```python
from build123d import *

# Parameters (mm, degrees)
SZKIC1_R                    = 2.25
DODANIE_WYCI_GNI_CIE1_DEPTH = 4


with BuildPart() as part:
    # Szkic1 → Dodanie-wyciągnięcie1 (new body)
    with BuildSketch(Plane.XY):
        with BuildLine():
            Line((-0.65, 5.460113222), (-0.65, 4.452808103))
            ThreePointArc((-0.65, 4.452808103), (-1.076920489, 4.369238178), (-1.493776689, 4.244835827))
            Line((-1.493776689, 4.244835827), (-1.96189472, 5.136760215))
            Line((-1.96189472, 5.136760215), (-2.706408708, 5.9097675))
            Line((-2.706408708, 5.9097675), (-3.326227926, 5.58446128))
            Line((-3.326227926, 5.58446128), (-3.112987553, 4.532620091))
            Line((-3.112987553, 4.532620091), (-2.644869523, 3.640695704))
            ThreePointArc((-2.644869523, 3.640695704), (-2.984051962, 3.368298367), (-3.295347141, 3.06442282))
            Line((-3.295347141, 3.06442282), (-4.124343002, 3.636637347))
            Line((-4.124343002, 3.636637347), (-5.142811797, 3.975108403))
            Line((-5.142811797, 3.975108403), (-5.54045712, 3.399019697))
            Line((-5.54045712, 3.399019697), (-4.862827173, 2.566758322))
            Line((-4.862827173, 2.566758322), (-4.033831312, 1.994543794))
            ThreePointArc((-4.033831312, 1.994543794), (-4.207573092, 1.595721992), (-4.341993276, 1.181987475))
            Line((-4.341993276, 1.181987475), (-5.341954007, 1.30340469))
            Line((-5.341954007, 1.30340469), (-6.401058681, 1.129799877))
            Line((-6.401058681, 1.129799877), (-6.485434357, 0.434903665))
            Line((-6.485434357, 0.434903665), (-5.498651691, 0.012883153))
            Line((-5.498651691, 0.012883153), (-4.49869096, -0.108534062))
            ThreePointArc((-4.49869096, -0.108534062), (-4.467189933, -0.542415061), (-4.393941078, -0.971226957))
            Line((-4.393941078, -0.971226957), (-5.335787726, -1.328422275))
            Line((-5.335787726, -1.328422275), (-6.192900162, -1.974332186))
            Line((-6.192900162, -1.974332186), (-5.944676741, -2.628843556))
            Line((-5.944676741, -2.628843556), (-4.874801373, -2.54394339))
            Line((-4.874801373, -2.54394339), (-3.932954725, -2.186748072))
            ThreePointArc((-3.932954725, -2.186748072), (-3.703427397, -2.55629136), (-3.439289932, -2.901944997))
            Line((-3.439289932, -2.901944997), (-4.10725678, -3.655923705))
            Line((-4.10725678, -3.655923705), (-4.566022849, -4.626168538))
            Line((-4.566022849, -4.626168538), (-4.042065325, -5.090354399))
            Line((-4.042065325, -5.090354399), (-3.134192808, -4.517983161))
            Line((-3.134192808, -4.517983161), (-2.466225959, -3.764004452))
            ThreePointArc((-2.466225959, -3.764004452), (-2.091254274, -3.984552115), (-1.69673891, -4.16786241))
            Line((-1.69673891, -4.16786241), (-1.937802804, -5.145897073))
            Line((-1.937802804, -5.145897073), (-1.893124727, -6.21820543))
            Line((-1.893124727, -6.21820543), (-1.213465455, -6.385726395))
            Line((-1.213465455, -6.385726395), (-0.675578441, -5.457007437))
            Line((-0.675578441, -5.457007437), (-0.434514548, -4.478972774))
            ThreePointArc((-0.434514548, -4.478972774), (0, -4.5), (0.434514548, -4.478972774))
            Line((0.434514548, -4.478972774), (0.675578441, -5.457007437))
            Line((0.675578441, -5.457007437), (1.213465455, -6.385726395))
            Line((1.213465455, -6.385726395), (1.893124727, -6.21820543))
            Line((1.893124727, -6.21820543), (1.937802804, -5.145897073))
            Line((1.937802804, -5.145897073), (1.69673891, -4.16786241))
            ThreePointArc((1.69673891, -4.16786241), (2.091254274, -3.984552115), (2.466225959, -3.764004452))
            Line((2.466225959, -3.764004452), (3.134192808, -4.517983161))
            Line((3.134192808, -4.517983161), (4.042065325, -5.090354399))
            Line((4.042065325, -5.090354399), (4.566022849, -4.626168538))
            Line((4.566022849, -4.626168538), (4.10725678, -3.655923705))
            Line((4.10725678, -3.655923705), (3.439289932, -2.901944997))
            ThreePointArc((3.439289932, -2.901944997), (3.703427397, -2.55629136), (3.932954725, -2.186748072))
            Line((3.932954725, -2.186748072), (4.874801373, -2.54394339))
            Line((4.874801373, -2.54394339), (5.944676741, -2.628843556))
            Line((5.944676741, -2.628843556), (6.192900162, -1.974332186))
            Line((6.192900162, -1.974332186), (5.335787726, -1.328422275))
            Line((5.335787726, -1.328422275), (4.393941078, -0.971226957))
            ThreePointArc((4.393941078, -0.971226957), (4.467189933, -0.542415061), (4.49869096, -0.108534062))
            Line((4.49869096, -0.108534062), (5.498651691, 0.012883153))
            Line((5.498651691, 0.012883153), (6.485434357, 0.434903665))
            Line((6.485434357, 0.434903665), (6.401058681, 1.129799877))
            Line((6.401058681, 1.129799877), (5.341954007, 1.30340469))
            Line((5.341954007, 1.30340469), (4.341993276, 1.181987475))
            ThreePointArc((4.341993276, 1.181987475), (4.207573092, 1.595721992), (4.033831312, 1.994543794))
            Line((4.033831312, 1.994543794), (4.862827173, 2.566758322))
            Line((4.862827173, 2.566758322), (5.54045712, 3.399019697))
            Line((5.54045712, 3.399019697), (5.142811797, 3.975108403))
            Line((5.142811797, 3.975108403), (4.124343002, 3.636637347))
            Line((4.124343002, 3.636637347), (3.295347141, 3.06442282))
            ThreePointArc((3.295347141, 3.06442282), (2.984051962, 3.368298367), (2.644869523, 3.640695704))
            Line((2.644869523, 3.640695704), (3.112987553, 4.532620091))
            Line((3.112987553, 4.532620091), (3.326227926, 5.58446128))
            Line((3.326227926, 5.58446128), (2.706408708, 5.9097675))
            Line((2.706408708, 5.9097675), (1.96189472, 5.136760215))
            Line((1.96189472, 5.136760215), (1.493776689, 4.244835827))
            ThreePointArc((1.493776689, 4.244835827), (1.076920489, 4.369238178), (0.65, 4.452808103))
            Line((0.65, 4.452808103), (0.65, 5.460113222))
            Line((0.65, 5.460113222), (0.35, 6.490570083))
            Line((0.35, 6.490570083), (-0.35, 6.490570083))
            Line((-0.35, 6.490570083), (-0.65, 5.460113222))
        make_face()
        Circle(SZKIC1_R, mode=Mode.SUBTRACT)
    extrude(amount=DODANIE_WYCI_GNI_CIE1_DEPTH)


solid = part.part
```
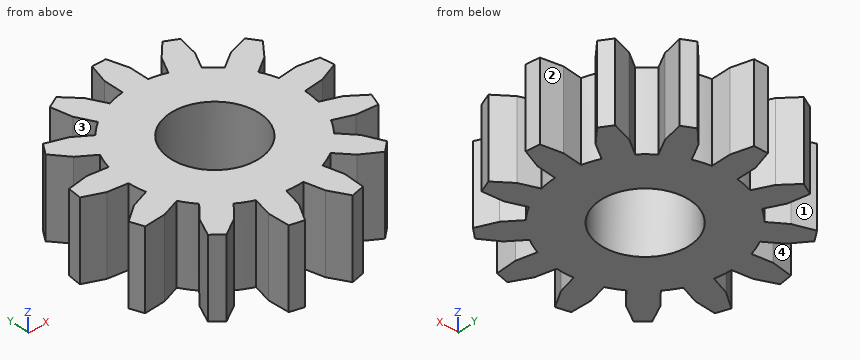
Can you work these out from the model? Positions are in its coordinate system, mm. Face numbers are marked on the shaded views. A direction names the side the tool comes from. Round coordinates to 2 decimals unless told otherwise and drop trailing zeros. Loops run counter-clockwise (first coordinate to the right, second up) from the corner with the lowest first, then second, coordinate; pieces in that order, holes last. Notation, with made-up numbers: (17.25, -10) -> (54.25, -10) arc R11 ccw to (54.25, 0) -> close; hole circle Ø8 at (-17.75, -12). An arc over 180 degrees is marked (long way). Answer in a Markdown table with one row per item.
Item 1: On a 3-axis mill with a long thin cutter (end or side, diameter ignored), from which of +Z, -Z, +X, -X, +Y, -Y can I reach the whole of each face in a straight line? I mean the marked faces 1, 2, 3 and 4. Say none if no direction works.
Answer block:
| item | result |
|---|---|
| face 1 | +Z, -Z, +Y |
| face 2 | +Z, -Z, +X |
| face 3 | +Z, -Z |
| face 4 | +Z, -Z, -X |
Item 2: Suppose I cut it at A-A, the plane x = 0. List the corners of the cut face in (y, z) for me, plus the area to 3 significant figures.
Answer block:
| item | result |
|---|---|
| outline | (-4.5, 0) -> (-2.25, 0) -> (-2.25, 4) -> (-4.5, 4) -> close; (2.25, 0) -> (6.49, 0) -> (6.49, 4) -> (2.25, 4) -> close |
| area | 26.0 mm² |
Item 3: If I drill on probe 1 along Y at (x, z) = (0, 1.8); probe 2 along X at (y, z) = (4.5, 3.65); probe 3 along X at (y, z) = (-4.75, 1.85), over which ranges is the centre line in solid material (lowest first)?
Answer block:
| item | result |
|---|---|
| probe 1 | -4.5 to -2.25, 2.25 to 6.49 |
| probe 2 | -3.1 to -1.63, -0.65 to 0.65, 1.63 to 3.1 |
| probe 3 | -4.43 to -3.5, -1.84 to -0.5, 0.5 to 1.84, 3.5 to 4.43 |
Item 4: Will this pin go through, and if not, where does the flat tip stop? P1, Ø1.1, axis at y = 5, z = 3, coming from the +X side.
Answer block:
| item | result |
|---|---|
| P1 | x = 3.32 |
